Verification items for the finished model (mm, model axes). Face numbers are marked on the shaded views. A direction names the side the tool comes from. Coordinates: 2 decimals unless noted, no trailing zeros. Order: outer loops, then holes, each group sorted by start corner. A loop starts at its lowest first (then second) coordinate and runs counter-clockwise, first axis right, second up. Notation, with made-up numbers: M 89.5,46 L 143.5,46 A22 ccw 143.5,72 Z; hole C 4.5,-25.75 d3. An arc over 180 degrees is marked long. Use one line per item in the form item = value. Start each with the question number.
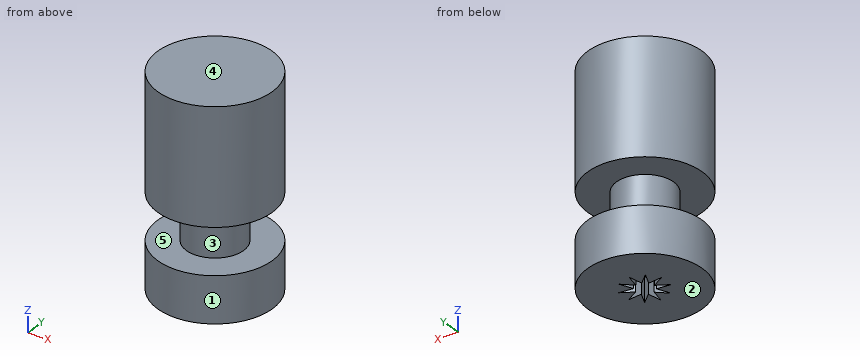
Autodesk Fusion 360 part; units mm, degrees
cylinder "CylinderPrimitive1" add diameter 5 height 2 placed x (1, 0, 0) y (0, 1, 0) z (0, 0, 1) at (0, 0, 0)
cylinder "CylinderPrimitive2" add diameter 2.5 height 2 placed x (1, 0, 0) y (0, 1, 0) z (0, 0, 1) at (0, 0, 2)
cylinder "CylinderPrimitive3" add diameter 5 height 5 placed x (1, 0, 0) y (0, 1, 0) z (0, 0, 1) at (0, 0, 4)
hole "Hole1" at (0, 0, 0) direction (0, 0, 1) diameter 2 depth 1 tip angle 180
sketch "Sketch5" plane through (0, 0, 1) normal (0, 0, -1) x (1, 0, 0)
  circle A0 centre (0, 0) radius 1
  line L0 (-1, 0.0018) -> (-0.4102, 0.0018)
  line L1 (-0.4102, 0.0018) -> (-1.1, 0.4)
  line L2 (-0.4102, 0.0018) -> (-0.9506, -0.3103)
  line L3 (-0.4102, 0.0018) -> (-1.1146, 0.0018) construction
  dimension "d10" = 30
  dimension "d11" = 30
extrude "Extrude1" add sketch "Sketch5" along normal blind 1 contours A0 L0 L1
extrude "Extrude2" add sketch "Sketch5" along normal blind 1 contours A0 L0 L2
pattern_circular "C-Pattern1" count 10 over 360 about axis through (0, 0, 2) along (0, 0, 1) of "Extrude1", "Extrude2"
1. Release check for a two-part mould opening along Z. For the marked faces 1, 2 and 3 record: pulls with the +Z half, pulls with the -Z half, needs draft (parallel to the pull), parting line crosses it, or undercut.
2. Cross-section at B-B on x = 1.7. Enter the section's corners in (y, z).
3. Cross-section at A-A on y = 2.05. Enter the section's corners in (x, z).
4. Depth check by flat-ended pin: P1, Ø2, axis at x = 1.5, z = 3.5, coming from the -Y side; P2, Ø1.5, axis at x = 2, z = 7.5, coming from the +Y side; P3, Ø2, axis at x = -2, z = 1, coming from the -Y side. Enter the tip coordinate at first touch or a pass-through.
5. Tool access check on the marked faces 4 and 5. Record the directions out of +Z, -Z, +X, -X, +Y, -Y that give a thin tool (end or side, any length) a straight path to the whole face; none if there is none.
6. Cross-section at C-C on y = -0.65. Enter the section's corners in (x, z).
7. Material ranges on line 1 along Z through (x, y) = (-1.15, -1.7); line 2 along Y through (x, z) = (0.05, 2.5); line 3 along X through (y, z) = (-0.55, 4.5), recorded low to high.
8. Cross-section at D-D on x = -1.15. Enter the section's corners in (y, z).
Final values:
q1.face_1 = needs draft
q1.face_2 = pulls with the -Z half
q1.face_3 = undercut
q2.outline = M -1.83,0 L 1.83,0 L 1.83,2 L -1.83,2 Z; M -1.83,4 L 1.83,4 L 1.83,9 L -1.83,9 Z
q3.outline = M -1.43,0 L 1.43,0 L 1.43,2 L -1.43,2 Z; M -1.43,4 L 1.43,4 L 1.43,9 L -1.43,9 Z
q4.P1 = -2.42
q4.P2 = 2.17
q4.P3 = -2.29
q5.face_4 = +Z, +X, -X, +Y, -Y
q5.face_5 = none
q6.outline = M -2.41,0 L -0.51,0 L -0.51,1 L -0.41,1 L -0.41,0 L -0.07,0 L -0.07,1 L 0.07,1 L 0.07,0 L 0.42,0 L 0.42,1 L 0.52,1 L 0.52,0 L 2.41,0 L 2.41,2 L 1.07,2 L 1.07,4 L 2.41,4 L 2.41,9 L -2.41,9 L -2.41,4 L -1.07,4 L -1.07,2 L -2.41,2 Z
q7.line_1 = 0 to 2, 4 to 9
q7.line_2 = -1.25 to 1.25
q7.line_3 = -2.44 to 2.44
q8.outline = M -2.22,0 L 2.22,0 L 2.22,2 L 0.49,2 L 0.49,4 L 2.22,4 L 2.22,9 L -2.22,9 L -2.22,4 L -0.49,4 L -0.49,2 L -2.22,2 Z
